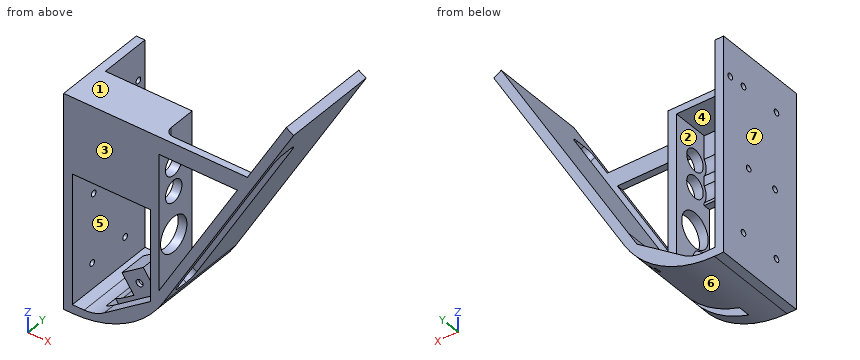
```python
from build123d import *

# Parameters (mm, degrees)
BOSS_EXTRUDE3_DEPTH     = 55
FILLET1_R               = 60
SKETCH4_W               = 15
SKETCH4_H               = 16
BOSS_EXTRUDE4_DEPTH     = 12
CUT_EXTRUDE1_DEPTH      = 20
CUT_EXTRUDE1_DEPTH_BACK = 14
SKETCH5_W               = 40
SKETCH5_H               = 7
CUT_EXTRUDE2_DEPTH      = 14
SKETCH7_R               = 2
CUT_EXTRUDE3_DEPTH      = 2
CUT_EXTRUDE4_DEPTH      = 30
SKETCH9_R               = 10
SKETCH9_R_2             = 6.25
CUT_EXTRUDE5_DEPTH      = 5
SKETCH10_W              = 120
SKETCH10_H              = 15
CUT_EXTRUDE6_DEPTH      = 5
SKETCH11_W              = 4
SKETCH11_H              = 25
BOSS_EXTRUDE5_DEPTH     = 45
FILLET3_R               = 20
BOSS_EXTRUDE6_REACH     = 190.434
SKETCH12_W              = 10
SKETCH12_H              = 4
SKETCH13_W              = 40
SKETCH13_H              = 4
BOSS_EXTRUDE7_DEPTH     = 45
FILLET4_R               = 5
FILLET5_R               = 5
CUT_EXTRUDE7_DEPTH      = 45
SKETCH16_R              = 1.75
CUT_EXTRUDE8_DEPTH      = 5
SKETCH15_R              = 1.75
CUT_EXTRUDE9_DEPTH      = 5
CUT_EXTRUDE10_REACH     = 216.345
SKETCH17_R              = 1.75
SKETCH17_R_2            = 1


with BuildPart() as part:
    # Sketch3 → Boss-Extrude3 (new body)
    with BuildSketch(Plane(origin=(0, 0, 0), x_dir=(1, 0, 0), z_dir=(0, 1, 0))):
        Polygon((128.169872981, -162.7146997), (55, -35.980762114), (55, -124), (50, -124), (50, -27.320508076), (18.123010882, -5), (5, -5), (5, -124), (0, -124), (0, 0), (40, 0), (132.5, -160.2146997), align=None)
    extrude(amount=BOSS_EXTRUDE3_DEPTH)

    # Fillet1
    fillet1_edges = [part.edges().sort_by_distance(p)[0] for p in [
        (40, 27.5, 0),
    ]]
    fillet(fillet1_edges, radius=FILLET1_R)

    # Sketch4 → Boss-Extrude4 (add)
    with BuildSketch(Plane(origin=(3.613056499, 0, -5.159979438), x_dir=(0.8191520442889911, 0, 0.5735764363510469), z_dir=(-0.5735764363510469, 0, 0.8191520442889911))):
        with Locations((39.128001876, 22.366188336)):
            Rectangle(SKETCH4_W, SKETCH4_H)
    extrude(amount=BOSS_EXTRUDE4_DEPTH)

    # Sketch5 → Cut-Extrude1 (cut, two sides: drawn at the far end of the back side and taken through both)
    with BuildSketch(Plane(origin=(3.613056499, 0, -5.159979438), x_dir=(0.8191520442889911, 0, 0.5735764363510469), z_dir=(-0.5735764363510469, 0, 0.8191520442889911)).offset(-CUT_EXTRUDE1_DEPTH_BACK)):
        with Locations((39.128001876, 10.866188336)):
            Rectangle(SKETCH5_W, SKETCH5_H)
    extrude(amount=CUT_EXTRUDE1_DEPTH + CUT_EXTRUDE1_DEPTH_BACK, mode=Mode.SUBTRACT)

    # Sketch6 → Cut-Extrude2 (cut)
    with BuildSketch(Plane(origin=(0, 30.366188336, 0), x_dir=(1, 0, 0), z_dir=(0, 1, 0))):
        Polygon((31.077587777, -14.070892396), (25.28446577, -22.344328043), (34.458968666, -28.76838413), (40.252090673, -20.494948483), align=None)
    extrude(amount=-CUT_EXTRUDE2_DEPTH, mode=Mode.SUBTRACT)

    # Sketch7 → Cut-Extrude3 (cut)
    with BuildSketch(Plane(origin=(0, 16.366188336, 0), x_dir=(1, 0, 0), z_dir=(0, 1, 0))):
        with Locations(Location((32.768278221, -21.419638263, 0), (0, 0, 270))):
            Circle(SKETCH7_R)
    extrude(amount=-CUT_EXTRUDE3_DEPTH, mode=Mode.SUBTRACT)

    # Sketch8 → Cut-Extrude4 (cut)
    with BuildSketch(Plane(origin=(0, 55, 0), x_dir=(1, 0, 0), z_dir=(0, 1, 0))):
        Polygon((55, -35.980762114), (50, -27.320508076), (50, -124), (55, -124), align=None)
    extrude(amount=-CUT_EXTRUDE4_DEPTH, mode=Mode.SUBTRACT)

    # Sketch9 → Cut-Extrude5 (cut)
    with BuildSketch(Plane.ZY.offset(-50)):
        with Locations((61.598678321, 11)):
            Circle(SKETCH9_R)
        with Locations((86.385123427, 11)):
            Circle(SKETCH9_R_2)
        with Locations((101.700022006, 11)):
            Circle(SKETCH9_R_2)
    extrude(amount=-CUT_EXTRUDE5_DEPTH, mode=Mode.SUBTRACT)

    # Sketch10 → Cut-Extrude6 (cut)
    with BuildSketch(Plane(origin=(30, 0, -17.320508076), x_dir=(-0.5000000000000047, 0, -0.866025403784436), z_dir=(0.866025403784436, 0, -0.5000000000000047))):
        with Locations((-119.641016151, 11.5)):
            Rectangle(SKETCH10_W, SKETCH10_H)
    extrude(amount=-CUT_EXTRUDE6_DEPTH, mode=Mode.SUBTRACT)

    # Sketch11 → Boss-Extrude5 (add)
    with BuildSketch(Plane.ZY.offset(-50)):
        with Locations((122, 12.5)):
            Rectangle(SKETCH11_W, SKETCH11_H)
    extrude(amount=BOSS_EXTRUDE5_DEPTH)

    # Fillet3
    # the kernel refuses this fillet: 20 mm, written as the material it adds along each edge
    with BuildSketch(Plane(origin=(18.123010882, 0, 5), x_dir=(-1, 0, 0), z_dir=(0, 1, 0))) as fillet3_piece_1_section:
        with BuildLine():
            CenterArc((FILLET3_R * 0.315298788879, FILLET3_R), FILLET3_R, 235, 35)
            Line((-FILLET3_R * 0.258277647472, FILLET3_R * 0.180847955711), (0, 0))
            Line((0, 0), (FILLET3_R * 0.315298788879, 0))
        make_face()
    fillet3_piece_1 = extrude(amount=55, mode=Mode.PRIVATE)
    fillet3_piece_1 = split(fillet3_piece_1, bisect_by=Plane(origin=(18.647698148, 3.683094168, 6.716980636), z_dir=(-0.8191520442889912, 0, -0.5735764363510469)), keep=Keep.TOP, mode=Mode.PRIVATE)
    fillet3_piece_1 = split(fillet3_piece_1, bisect_by=Plane(origin=(16.403340896, 7.366188336, 5.14546477), z_dir=(0, -1, 0)), keep=Keep.TOP, mode=Mode.PRIVATE)
    add(fillet3_piece_1)
    with BuildSketch(Plane(origin=(18.123010882, 0, 5), x_dir=(-1, 0, 0), z_dir=(0, 1, 0))) as fillet3_piece_2_section:
        with BuildLine():
            CenterArc((FILLET3_R * 0.315298788879, FILLET3_R), FILLET3_R, 235, 35)
            Line((-FILLET3_R * 0.258277647472, FILLET3_R * 0.180847955711), (0, 0))
            Line((0, 0), (FILLET3_R * 0.315298788879, 0))
        make_face()
    fillet3_piece_2 = extrude(amount=55, mode=Mode.PRIVATE)
    fillet3_piece_2 = split(fillet3_piece_2, bisect_by=Plane(origin=(19.32323837, 3.683094168, 5.752209215), z_dir=(0.8191520442889912, 0, 0.5735764363510469)), keep=Keep.TOP, mode=Mode.PRIVATE)
    fillet3_piece_2 = split(fillet3_piece_2, bisect_by=Plane(origin=(20.990357579, 7.366188336, 6.919538653), z_dir=(0, -1, 0)), keep=Keep.TOP, mode=Mode.PRIVATE)
    add(fillet3_piece_2)
    with BuildSketch(Plane(origin=(18.123010882, 0, 5), x_dir=(-1, 0, 0), z_dir=(0, 1, 0))) as fillet3_piece_3_section:
        with BuildLine():
            CenterArc((FILLET3_R * 0.315298788879, FILLET3_R), FILLET3_R, 235, 35)
            Line((-FILLET3_R * 0.258277647472, FILLET3_R * 0.180847955711), (0, 0))
            Line((0, 0), (FILLET3_R * 0.315298788879, 0))
        make_face()
    fillet3_piece_3 = extrude(amount=55, mode=Mode.PRIVATE)
    fillet3_piece_3 = split(fillet3_piece_3, bisect_by=Plane(origin=(16.403340896, 14.366188336, 5.14546477), z_dir=(0, -1, 0)), keep=Keep.TOP, mode=Mode.PRIVATE)
    fillet3_piece_3 = split(fillet3_piece_3, bisect_by=Plane(origin=(18.647698148, 10.866188336, 6.716980636), z_dir=(-0.8191520442889912, 0, -0.5735764363510469)), keep=Keep.TOP, mode=Mode.PRIVATE)
    fillet3_piece_3 = split(fillet3_piece_3, bisect_by=Plane(origin=(16.403340896, 7.366188336, 5.14546477), z_dir=(0, 1, 0)), keep=Keep.TOP, mode=Mode.PRIVATE)
    add(fillet3_piece_3)
    with BuildSketch(Plane(origin=(18.123010882, 0, 5), x_dir=(-1, 0, 0), z_dir=(0, 1, 0))) as fillet3_piece_4_section:
        with BuildLine():
            CenterArc((FILLET3_R * 0.315298788879, FILLET3_R), FILLET3_R, 235, 35)
            Line((-FILLET3_R * 0.258277647472, FILLET3_R * 0.180847955711), (0, 0))
            Line((0, 0), (FILLET3_R * 0.315298788879, 0))
        make_face()
    fillet3_piece_4 = extrude(amount=55, mode=Mode.PRIVATE)
    fillet3_piece_4 = split(fillet3_piece_4, bisect_by=Plane(origin=(16.403340896, 14.366188336, 5.14546477), z_dir=(0, 1, 0)), keep=Keep.TOP, mode=Mode.PRIVATE)
    fillet3_piece_4 = split(fillet3_piece_4, bisect_by=Plane(origin=(18.647698148, 34.683094168, 6.716980636), z_dir=(-0.8191520442889912, 0, -0.5735764363510469)), keep=Keep.TOP, mode=Mode.PRIVATE)
    add(fillet3_piece_4)
    with BuildSketch(Plane(origin=(18.123010882, 0, 5), x_dir=(-1, 0, 0), z_dir=(0, 1, 0))) as fillet3_piece_5_section:
        with BuildLine():
            CenterArc((FILLET3_R * 0.315298788879, FILLET3_R), FILLET3_R, 235, 35)
            Line((-FILLET3_R * 0.258277647472, FILLET3_R * 0.180847955711), (0, 0))
            Line((0, 0), (FILLET3_R * 0.315298788879, 0))
        make_face()
    fillet3_piece_5 = extrude(amount=55, mode=Mode.PRIVATE)
    fillet3_piece_5 = split(fillet3_piece_5, bisect_by=Plane(origin=(20.990357579, 14.366188336, 6.919538653), z_dir=(0, 1, 0)), keep=Keep.TOP, mode=Mode.PRIVATE)
    fillet3_piece_5 = split(fillet3_piece_5, bisect_by=Plane(origin=(19.32323837, 34.683094168, 5.752209215), z_dir=(0.8191520442889912, 0, 0.5735764363510469)), keep=Keep.TOP, mode=Mode.PRIVATE)
    add(fillet3_piece_5)

    # Boss-Extrude6: up to this plane
    boss_extrude6_end = Plane(origin=(128.169872981, 55, 162.7146997), z_dir=(-0.8660254037844362, 0, 0.5000000000000044))
    # Sketch12 → Boss-Extrude6 (add, up to the surface)
    with BuildSketch(Plane(origin=(55, 0, 0), x_dir=(0, 0, -1), z_dir=(1, 0, 0)), mode=Mode.PRIVATE) as boss_extrude6_sk1:
        with Locations((-119, 2)):
            Rectangle(SKETCH12_W, SKETCH12_H)
    boss_extrude6_tool1 = split(extrude(boss_extrude6_sk1.sketch, amount=BOSS_EXTRUDE6_REACH, mode=Mode.PRIVATE), bisect_by=boss_extrude6_end, keep=Keep.BOTH, mode=Mode.PRIVATE)
    add(boss_extrude6_tool1.solids().sort_by_distance((55, 2, 119))[0])

    # Sketch13 → Boss-Extrude7 (add)
    with BuildSketch(Plane.ZY.offset(-50)):
        with Locations((100, 2)):
            Rectangle(SKETCH13_W, SKETCH13_H)
    extrude(amount=BOSS_EXTRUDE7_DEPTH)

    # Fillet4
    fillet4_edges = [part.edges().sort_by_distance(p)[0] for p in [
        (57.655444566, 4, 35.580127019),
        (57.655444566, 19, 35.580127019),
        (117.655444566, 19, 139.503175473),
        (117.655444566, 4, 139.503175473),
    ]]
    fillet(fillet4_edges, radius=FILLET4_R)

    # Fillet5
    fillet5_edges = [part.edges().sort_by_distance(p)[0] for p in [
        (55, 4, 119),
    ]]
    fillet(fillet5_edges, radius=FILLET5_R)

    # Sketch14 → Cut-Extrude7 (cut)
    with BuildSketch(Plane.ZY.offset(-50)):
        with BuildLine():
            ThreePointArc((94.042572717, 14.689643665), (77.885123427, 11), (94.042572717, 7.310356335))
            ThreePointArc((94.042572717, 7.310356335), (110.200022006, 11), (94.042572717, 14.689643665))
        make_face()
    extrude(amount=CUT_EXTRUDE7_DEPTH, mode=Mode.SUBTRACT)

    # Sketch16 → Cut-Extrude8 (cut)
    with BuildSketch(Plane.ZY):
        with Locations((59.208509529, 36.135781847)):
            Circle(SKETCH16_R)
        with Locations((59.208509529, 16.135781847)):
            Circle(SKETCH16_R)
        with Locations((103.718271361, 50.013687011)):
            Circle(SKETCH16_R)
    extrude(amount=-CUT_EXTRUDE8_DEPTH, mode=Mode.SUBTRACT)

    # Sketch15 → Cut-Extrude9 (cut)
    with BuildSketch(Plane.ZY):
        with Locations((104, 40)):
            Circle(SKETCH15_R)
        with Locations((104, 15)):
            Circle(SKETCH15_R)
        with Locations((20, 15)):
            Circle(SKETCH15_R)
        with Locations((20, 40)):
            Circle(SKETCH15_R)
    extrude(amount=-CUT_EXTRUDE9_DEPTH, mode=Mode.SUBTRACT)

    # Cut-Extrude10: up to this plane
    cut_extrude10_end = Plane(origin=(18.123010882, 55, 5), z_dir=(0.5735764363510469, 0, -0.8191520442889914))
    # Sketch17 → Cut-Extrude10 (cut, up to the surface)
    with BuildSketch(Plane(origin=(30, 0, -17.320508076), x_dir=(-0.5000000000000047, 0, -0.866025403784436), z_dir=(0.866025403784436, 0, -0.5000000000000047)), mode=Mode.PRIVATE) as cut_extrude10_sk1:
        with Locations((-34.202339372, 47.5)):
            Circle(SKETCH17_R)
    cut_extrude10_tool1 = split(extrude(cut_extrude10_sk1.sketch, amount=-CUT_EXTRUDE10_REACH, mode=Mode.PRIVATE), bisect_by=cut_extrude10_end, keep=Keep.BOTH, mode=Mode.PRIVATE)
    add(cut_extrude10_tool1.solids().sort_by_distance((47.10117, 47.5, 12.299587))[0], mode=Mode.SUBTRACT)
    # Sketch17 → Cut-Extrude10 (cut, up to the surface)
    with BuildSketch(Plane(origin=(30, 0, -17.320508076), x_dir=(-0.5000000000000047, 0, -0.866025403784436), z_dir=(0.866025403784436, 0, -0.5000000000000047)), mode=Mode.PRIVATE) as cut_extrude10_sk2:
        with Locations((-39.202339372, 47.5)):
            Circle(SKETCH17_R_2)
    cut_extrude10_tool2 = split(extrude(cut_extrude10_sk2.sketch, amount=-CUT_EXTRUDE10_REACH, mode=Mode.PRIVATE), bisect_by=cut_extrude10_end, keep=Keep.BOTH, mode=Mode.PRIVATE)
    add(cut_extrude10_tool2.solids().sort_by_distance((49.60117, 47.5, 16.629714))[0], mode=Mode.SUBTRACT)


solid = part.part
```
Model file for the job. Use its own axes, mm. Face numbers are marked on the shaded views. A direction names the side the tool comes from. Coordinates: 2 decimals unless noted, no trailing zeros. Write each loop counter-clockwise with the first axis right and the second up, starting at its lowest first coordinate (ties: lowest second). Pieces come first, ordered by that corner, then holes. Notation, with made-up numbers: (77, 23.5) - (133, 23.5) arc R16 ccw to (133, 53.5) - close; hole circle Ø7 at (-17.75, -37). An arc over 180 degrees is marked (long way). One line per item, written item: value. Start each with the question number.
1. Tool access for the marked faces 1, 2 and 3: list every direction of +Z, -Z, +X, -X, +Y, -Y with a clear straight run to the whole face (end or side of a thin tool).
2. Slice it at C-C (x = 15.5). Write the cut outline in (y, z).
3. Flat gauge pins, fed straight in: pin 1 (4 mm diameter, centred on y = 40, z = 20, fed in from +X); pin 2 (1.5 mm diameter, centred on y = 20.5, z = 68.5, fed in from +X); pin 3 (4 mm diameter, centred on y = 15, z = 104, fed in from +X); pin 4 (2.5 mm diameter, centred on x = 32.77, z = 21.42, fed in from +Y). Where does each tip first touch, or does it go through?
4. Slice it at D-D (z = 76). Write the cut outline in (x, y), plus the area to 3 significant figures.
5. Probe line 1 (Y direction, x = 2.65, z = 20); line 2 (Y direction, x = 2.75, z = 104); line 3 (X direction, y = 7, z = 51.5). List the from-to ranges inside material, lowest first. Write a range as from..to.
6. Slice it at A-A (y = 40). Write the cut outline in (x, z).
7. Slice it at B-B (y = 11). Count the separate pieces of the cut face and the enclosed holes in it, plus the area to 3 significant figures.
8. Mould opens along Z. For the marked faces 4, 5, 6 and 7 say: released by +Z, released by -Z, zero draft, split by the parting line, or undercut.
Answers below:
1. face 1: +Z, -X, +Y, -Y
1. face 2: +Y
1. face 3: +Z, -Z, +X, -X, -Y
2. outline: (0, 0.86) - (55, 0.86) - (55, 5.34) - (0, 5.34) - close; (0, 80) - (4, 80) - (4, 81.56) arc R8.5 cw to (4, 91.21) - (4, 96.88) arc R8.5 cw to (4, 106.52) - (4, 120) - (25, 120) - (25, 124) - (0, 124) - close
3. pin 1: stops at x = 51.79
3. pin 2: stops at x = 79.98
3. pin 3: stops at x = 55
3. pin 4: passes through
4. outline: (0, 0) - (5, 0) - (5, 55) - (0, 55) - close; (50, 0) - (55, 0) - (55, 25) - (50, 25) - close; (78.11, 0) - (83.88, 0) - (83.88, 4) - (78.11, 4) - close; (78.11, 19) - (83.88, 19) - (83.88, 55) - (78.11, 55) - close
4. area: 631 mm^2
5. line 1: y = 0..13.25, 16.75..38.25, 41.75..55
5. line 2: y = 0..13.25, 16.75..38.25, 41.75..48.29, 51.74..55
5. line 3: x = 0..5, 50..55
6. outline: (0, 0) - (5.36, 0) arc R60 ccw to (57.32, 30) - (132.5, 160.21) - (128.17, 162.71) - (50, 27.32) - (23.29, 8.62) arc R20 cw to (11.82, 5) - (5, 5) - (5, 18.25) - (0, 18.25) - close; (0, 21.75) - (5, 21.75) - (5, 102.25) - (0, 102.25) - close; (0, 105.75) - (5, 105.75) - (5, 124) - (0, 124) - close
7. separate pieces: 5
7. enclosed holes: 0
7. area: 1,280 mm^2
8. face 4: undercut
8. face 5: undercut
8. face 6: released by -Z
8. face 7: zero draft
